from build123d import *

# Parameters (mm, degrees)
EXTRUDE_1_DEPTH = 110
M10X1_0_1_D     = 9
M10X1_0_1_DEPTH = 23
M10X1_0_1_TIP   = 2.703872786


with BuildPart() as part:
    # 草图1 → 凸台-拉伸1 (new, symmetric)
    with BuildSketch(Plane.XY):
        with BuildLine():
            Line((-21, 40), (21, 40))
            ThreePointArc((21, 40), (34.435028843, 34.435028843), (40, 21))
            Line((40, 21), (40, -21))
            ThreePointArc((40, -21), (34.435028843, -34.435028843), (21, -40))
            Line((21, -40), (-21, -40))
            ThreePointArc((-21, -40), (-34.435028843, -34.435028843), (-40, -21))
            Line((-40, -21), (-40, 21))
            ThreePointArc((-40, 21), (-34.435028843, 34.435028843), (-21, 40))
        make_face()
        with BuildLine():
            Line((-32, 21), (-32, -21))
            ThreePointArc((-32, -21), (-28.778174593, -28.778174593), (-21, -32))
            Line((-21, -32), (21, -32))
            ThreePointArc((21, -32), (28.778174593, -28.778174593), (32, -21))
            Line((32, -21), (32, 21))
            ThreePointArc((32, 21), (28.778174593, 28.778174593), (21, 32))
            Line((21, 32), (-21, 32))
            ThreePointArc((-21, 32), (-28.778174593, 28.778174593), (-32, 21))
        make_face(mode=Mode.SUBTRACT)
    extrude(amount=EXTRUDE_1_DEPTH, both=True)

    # M10x1.0 螺纹孔1
    with Locations(Plane(origin=(0, -40, 0), x_dir=(-1, 0, 0), z_dir=(0, -1, 0))):
        with Locations((0, 0)):
            Hole(M10X1_0_1_D / 2, depth=M10X1_0_1_DEPTH)
            with Locations((0, 0, -(M10X1_0_1_DEPTH + M10X1_0_1_TIP / 2))):  # 118° drill point
                Cone(0, M10X1_0_1_D / 2, M10X1_0_1_TIP, mode=Mode.SUBTRACT)


solid = part.part
Design review of the part built by this model. Coordinates are the model's own, in mm. A direction names the side the tool comes from. Round coordinates to 2 decimals unless told otherwise and drop trailing zeros. Write each loop counter-clockwise with the first axis right and the second up, starting at its lowest first coordinate (ties: lowest second). Pieces come first, ordered by that corner, then holes.
Item 1: For faces 5 (the flat face through (40, 0, 2)), 6 (the cylindrical face through (-0.59, -35.94, -4.46)), 7 (the flat face through (-32, 0, 2)), list the 3-axis set-ups (+Z, -Z, +X, -X, +Y, -Y) from which the entire face can be reached by the end or side of a thin tool; tool diameter is ignored.
Item 2: Consider section B-B on y = 12. Give the boundary of the cut face in (x, z), and give its area (3 significant figures).
Item 3: Draft analysis for pull direction Y (two halves, no side actions). For faces 1 (the flat face through (-40, 0, 2)), 2 (the flat face through (5, -40, 2)), 3 (the flat face through (32, 0, 2)), 4 (the cylindrical face through (28.863, 28.692, 1.54)), state which applies: released by +Y, released by -Y, zero draft, split by the parting line, or undercut.
Item 4: Wall thickness on L1, parallel to X at y = -16.5, z = -36.5; L2, parallel to Z at x = 0, y = -37: over which ranges is each line inside the solid? List them lowest first.
Item 5: Consider section A-A on x = 0. Give the boundary of the cut face in (y, z), and give its area (3 significant figures).
Item 6: For pin 1 Ø2 at (y, z) = (25, 26.5) entering from -X, flat-tipped, find the tip position at first contact; note if it passes through.
Item 7: Consider section C-C on z = -15. Give the boundary of the cut face in (x, y), and give its area (3 significant figures).
Check values:
1. face 5: +Z, -Z, +X, +Y, -Y
1. face 6: -Y
1. face 7: +Z, -Z
2. outline: (-40, -110) - (-32, -110) - (-32, 110) - (-40, 110) - close; (32, -110) - (40, -110) - (40, 110) - (32, 110) - close
2. area: 3,520 mm2
3. face 1: zero draft
3. face 2: released by -Y
3. face 3: undercut
3. face 4: undercut
4. L1: x = -40 to -32, 32 to 40
4. L2: z = -110 to -4.5, 4.5 to 110
5. outline: (-40, -110) - (-32, -110) - (-32, -4.5) - (-40, -4.5) - close; (-40, 4.5) - (-32, 4.5) - (-32, 110) - (-40, 110) - close; (32, -110) - (40, -110) - (40, 110) - (32, 110) - close
5. area: 3,450 mm2
6. pin 1: stops at x = -39.76
7. outline: (-40, -21) arc R19 ccw to (-21, -40) - (21, -40) arc R19 ccw to (40, -21) - (40, 21) arc R19 ccw to (21, 40) - (-21, 40) arc R19 ccw to (-40, 21) - close; hole (-32, -21) arc R11 ccw to (-21, -32) - (21, -32) arc R11 ccw to (32, -21) - (32, 21) arc R11 ccw to (21, 32) - (-21, 32) arc R11 ccw to (-32, 21) - close
7. area: 2,100 mm2
